Input: part model. Units: mm. Frame: model coordinates. A direction names the side the tool comes from. Round coordinates to 2 decimals unless told otherwise and drop trailing zeros. Loops run counter-clockwise (first coordinate to the right, second up) from the corner with the lowest first, then second, coordinate; pieces in that order, holes last.
1) Ray query, line 1 along X through (y, z) = (12.5, -3.75); line 2 along X through (y, z) = (3.75, -8.75); line 3 along X through (y, z) = (8.5, -2.75). Return the intervals inside material, ascending.
2) Section D-D, the plane x = 16.5. Return loops of the section in (y, z), and give its area (3 significant figures).
3) Section A-A, the plane x = 97. Return loops of the section in (y, z), and give its area (3 significant figures).
4) First-contact query: pin 1 (5.5 mm diameter, centred on x = 55.5, z = -22, fed in from +Y); pin 2 (4 mm diameter, centred on x = 91.5, y = 9.5, fed in from +Z); pin 3 (5.5 mm diameter, centred on x = 16.5, y = 4, fed in from +Z); pin 4 (8 mm diameter, centred on x = 55, y = 11.5, fed in from +Z). Flat tips, straight axial feed; report the tip coordinate or a pass-through.
5) Section B-B, the plane z = -13.5. State how many separate pieces and enclosed holes the cut face has, and give its area (3 significant figures).
6) Access query for faces 1 (the face through (63, 5, -20)), 2 (the face through (100, 1, -23)), 3 (the face through (77, 8, -2)). Directions: +Z, -Z, +X, -X, +Y, -Y. A direction counts if a zero-diameter tool reaches every point of the face in a straight line with its end or side. Return the directions, or none.
7) Draft query along X for faces 4 (the face through (2, 3, -16)), 5 (the face through (30, 8, -15)), 6 (the face through (110, 18, -13)). Return one class per face: pulls with the +X half, pulls with the -X half, needs draft (parallel to the pull), parting line crosses it, or undercut.
from build123d import *

# Parameters (mm, degrees)
SKETCH1_W          = 110
SKETCH1_H          = 25
BASE_DEPTH         = 1
SKETCH10_W         = 5
SKETCH10_H         = 5
LEG1_DEPTH         = 4
LEG2_W             = 5
LEG2_H             = 5
LEG2E_DEPTH        = 6
LEG3_W             = 5
LEG3_H             = 5
LEG3E_DEPTH        = 8
LEG4_W             = 5
LEG4_H             = 5
LEG4E_DEPTH        = 10
LEG5_W             = 5
LEG5_H             = 5
LEG5E_DEPTH        = 12
LEG6_W             = 5
LEG6_H             = 5
LEG6E_DEPTH        = 14
LEG7_W             = 5
LEG7_H             = 5
LEG7E_DEPTH        = 16
LEG8_W             = 5
LEG8_H             = 5
LEG8E_DEPTH        = 18
SKETCH29_W         = 5
SKETCH29_H         = 2
BRIDGE1_DEPTH      = 8
SKETCH30_W         = 5
SKETCH30_H         = 2
BRIDGE2_DEPTH      = 9
SKETCH31_W         = 5
SKETCH31_H         = 2
BRIDGE3_DEPTH      = 10
SKETCH32_W         = 5
SKETCH32_H         = 2
BRIDGE4_DEPTH      = 11
SKETCH33_W         = 5
SKETCH33_H         = 2
BRIDGE5_DEPTH      = 12
SKETCH34_W         = 5
SKETCH34_H         = 2
BRIDGE6_DEPTH      = 13
SKETCH35_W         = 5
SKETCH35_H         = 2
BRIDGE7_DEPTH      = 14
SKETCH36_W         = 5
SKETCH36_H         = 2
BRIDGE8_DEPTH      = 15
CUT_EXTRUDE4_DEPTH = 115.232219623


with BuildPart() as part:
    # Sketch1 → Base (new body)
    with BuildSketch(Plane(origin=(0, 0, 0), x_dir=(1, 0, 0), z_dir=(0, 1, 0))):
        with Locations((55, 12.5)):
            Rectangle(SKETCH1_W, SKETCH1_H)
    extrude(amount=BASE_DEPTH)

    # Sketch10 → leg1 (add)
    with BuildSketch(Plane(origin=(0, 1, 0), x_dir=(1, 0, 0), z_dir=(0, 1, 0))):
        with Locations((2.5, 22.5)):
            Rectangle(SKETCH10_W, SKETCH10_H)
        with Locations((2.5, 9.5)):
            Rectangle(SKETCH10_W, SKETCH10_H)
    extrude(amount=LEG1_DEPTH)

    # leg2 → leg2e (add)
    with BuildSketch(Plane(origin=(0, 1, 0), x_dir=(1, 0, 0), z_dir=(0, 1, 0))):
        with Locations((17.5, 22.5)):
            Rectangle(LEG2_W, LEG2_H)
        with Locations((17.5, 8.5)):
            Rectangle(LEG2_W, LEG2_H)
    extrude(amount=LEG2E_DEPTH)

    # leg3 → leg3e (add)
    with BuildSketch(Plane(origin=(0, 1, 0), x_dir=(1, 0, 0), z_dir=(0, 1, 0))):
        with Locations((32.5, 22.5)):
            Rectangle(LEG3_W, LEG3_H)
        with Locations((32.5, 7.5)):
            Rectangle(LEG3_W, LEG3_H)
    extrude(amount=LEG3E_DEPTH)

    # leg4 → leg4e (add)
    with BuildSketch(Plane(origin=(0, 1, 0), x_dir=(1, 0, 0), z_dir=(0, 1, 0))):
        with Locations((47.5, 22.5)):
            Rectangle(LEG4_W, LEG4_H)
        with Locations((47.5, 6.5)):
            Rectangle(LEG4_W, LEG4_H)
    extrude(amount=LEG4E_DEPTH)

    # leg5 → leg5e (add)
    with BuildSketch(Plane(origin=(0, 1, 0), x_dir=(1, 0, 0), z_dir=(0, 1, 0))):
        with Locations((62.5, 22.5)):
            Rectangle(LEG5_W, LEG5_H)
        with Locations((62.5, 5.5)):
            Rectangle(LEG5_W, LEG5_H)
    extrude(amount=LEG5E_DEPTH)

    # leg6 → leg6e (add)
    with BuildSketch(Plane(origin=(0, 1, 0), x_dir=(1, 0, 0), z_dir=(0, 1, 0))):
        with Locations((77.5, 22.5)):
            Rectangle(LEG6_W, LEG6_H)
        with Locations((77.5, 4.5)):
            Rectangle(LEG6_W, LEG6_H)
    extrude(amount=LEG6E_DEPTH)

    # leg7 → leg7e (add)
    with BuildSketch(Plane(origin=(0, 1, 0), x_dir=(1, 0, 0), z_dir=(0, 1, 0))):
        with Locations((92.5, 22.5)):
            Rectangle(LEG7_W, LEG7_H)
        with Locations((92.5, 3.5)):
            Rectangle(LEG7_W, LEG7_H)
    extrude(amount=LEG7E_DEPTH)

    # leg8 → leg8e (add)
    with BuildSketch(Plane(origin=(0, 1, 0), x_dir=(1, 0, 0), z_dir=(0, 1, 0))):
        with Locations((107.5, 22.5)):
            Rectangle(LEG8_W, LEG8_H)
        with Locations((107.5, 2.5)):
            Rectangle(LEG8_W, LEG8_H)
    extrude(amount=LEG8E_DEPTH)

    # Sketch29 → bridge1 (add)
    with BuildSketch(Plane.XY.offset(-20)):
        with Locations((2.5, 4)):
            Rectangle(SKETCH29_W, SKETCH29_H)
    extrude(amount=BRIDGE1_DEPTH)

    # Sketch30 → bridge2 (add)
    with BuildSketch(Plane.XY.offset(-20)):
        with Locations((17.5, 6)):
            Rectangle(SKETCH30_W, SKETCH30_H)
    extrude(amount=BRIDGE2_DEPTH)

    # Sketch31 → bridge3 (add)
    with BuildSketch(Plane.XY.offset(-20)):
        with Locations((32.5, 8)):
            Rectangle(SKETCH31_W, SKETCH31_H)
    extrude(amount=BRIDGE3_DEPTH)

    # Sketch32 → bridge4 (add)
    with BuildSketch(Plane.XY.offset(-20)):
        with Locations((47.5, 10)):
            Rectangle(SKETCH32_W, SKETCH32_H)
    extrude(amount=BRIDGE4_DEPTH)

    # Sketch33 → bridge5 (add)
    with BuildSketch(Plane.XY.offset(-20)):
        with Locations((62.5, 12)):
            Rectangle(SKETCH33_W, SKETCH33_H)
    extrude(amount=BRIDGE5_DEPTH)

    # Sketch34 → bridge6 (add)
    with BuildSketch(Plane.XY.offset(-20)):
        with Locations((77.5, 14)):
            Rectangle(SKETCH34_W, SKETCH34_H)
    extrude(amount=BRIDGE6_DEPTH)

    # Sketch35 → bridge7 (add)
    with BuildSketch(Plane.XY.offset(-20)):
        with Locations((92.5, 16)):
            Rectangle(SKETCH35_W, SKETCH35_H)
    extrude(amount=BRIDGE7_DEPTH)

    # Sketch36 → bridge8 (add)
    with BuildSketch(Plane.XY.offset(-20)):
        with Locations((107.5, 18)):
            Rectangle(SKETCH36_W, SKETCH36_H)
    extrude(amount=BRIDGE8_DEPTH)

    # Sketch37 → Cut-Extrude4 (cut, through all)
    with BuildSketch(Plane(origin=(0, 1, 0), x_dir=(1, 0, 0), z_dir=(0, 1, 0))):
        Polygon((0, 20), (110, 20), (110, 5), (95, 5), (95, 6), (80, 6), (80, 7), (65, 7), (65, 8), (50, 8), (50, 9), (35, 9), (35, 10), (20, 10), (20, 11), (5, 11), (5, 12), (0, 12), align=None)
    extrude(amount=-CUT_EXTRUDE4_DEPTH, mode=Mode.SUBTRACT)


solid = part.part
Final values:
1. line 1: x = 60 to 65, 75 to 80, 90 to 95, 105 to 110
1. line 2: x = 0 to 5, 15 to 20, 30 to 35, 45 to 50
1. line 3: x = 75 to 80, 90 to 95, 105 to 110
2. outline: (0, -25) - (7, -25) - (7, -6) - (1, -6) - (1, 0) - (0, 0) - (0, -11) - (5, -11) - (5, -20) - (0, -20) - close
2. area: 94.0 mm2
3. outline: (0, -25) - (1, -25) - (1, -20) - (0, -20) - close; (0, -5) - (1, -5) - (1, 0) - (0, 0) - close
3. area: 10.0 mm2
4. pin 1: stops at y = 1
4. pin 2: stops at z = -1
4. pin 3: stops at z = -6
4. pin 4: passes through
5. separate pieces: 8
5. enclosed holes: 0
5. area: 80.0 mm2
6. face 1: +X, -Y
6. face 2: +Z, -Z, +Y
6. face 3: +Z, -X, +Y
7. face 4: needs draft
7. face 5: undercut
7. face 6: pulls with the +X half
